```python
from build123d import *

# Parameters (mm, degrees)
F0_W     = 100
F0_H     = 100
F1_DEPTH = 100
F2_R     = 10
F3_R     = 7.3330548606
F4_DEPTH = 5
F5_R     = 7.0099311872
F5_R_2   = 5.9405048223
F6_DEPTH = 18


# Not quite as in the source:
# - a fillet or chamfer that OpenCascade refuses, or shapes differently, is made with other operations: its cross-section is extruded or revolved along the edge and cut away or added


with BuildPart() as f1:
    # F0 (on Top) → F1 (new body)
    with BuildSketch(Plane.XY):
        Rectangle(F0_W, F0_H)
    extrude(amount=F1_DEPTH)

    # F2
    f2_edges = [f1.edges().sort_by_distance(p)[0] for p in [
        (-50, -50, 50),
        (0, -50, 0),
        (50, -50, 50),
        (-50, 0, 100),
        (0, 50, 100),
        (50, 0, 100),
        (0, -50, 100),
        (-50, 0, 0),
        (-50, 50, 50),
        (0, 50, 0),
        (50, 50, 50),
        (50, 0, 0),
    ]]
    fillet(f2_edges, radius=F2_R)

    # F3 (on face) → F4 (cut)
    with BuildSketch(Plane(origin=(-50, 0, 0), x_dir=(0, -1, 0), z_dir=(-1, 0, 0))):
        with Locations((1.8755461788, 50)):
            Circle(F3_R)
    extrude(amount=-F4_DEPTH, mode=Mode.SUBTRACT)

    # F5 (on face) → F6 (cut)
    with BuildSketch(Plane.YZ.offset(50)):
        with Locations((19.523344934, 76.1831775308)):
            Circle(F5_R)
        with Locations((-10.0353639573, 45.1647788286)):
            Circle(F5_R_2)
    extrude(amount=-F6_DEPTH, mode=Mode.SUBTRACT)

    # F7: fillet of radius 7.2426406871 on 5 edges, made by hand

    # F7_s1 → F7_t2 (revolve)
    with BuildSketch(Plane.XY.offset(50)):
        with BuildLine():
            ThreePointArc((-50, -9.2086010394), (-46.3818180141, -6.5771030138), (-45, -2.3219177396))
            Line((-45, -2.3219177396), (-45, -9.2086010394))
            Line((-45, -9.2086010394), (-50, -9.2086010394))
        make_face()
    revolve(axis=Axis((-45, -1.8755461788, 50), (-1, 0, 0)))


solid = f1.part
```
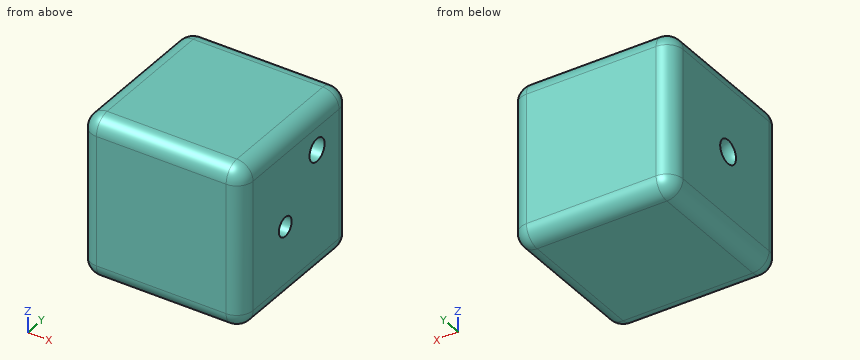
Read the model definition and answer for the solid it produces. Units are mm, in the model's axes. Give positions to 0.01 mm unless a question says otherwise; leave off trailing zeros. Order: outer loops, then holes, each group sorted by start corner. A loop starts at its lowest first (then second) coordinate and runs counter-clockwise, first axis right, second up. Notation, with made-up numbers: (49.5, 44.5) -> (53.5, 44.5) arc R30 ccw to (53.5, 71.5) -> close; hole circle Ø2 at (71.5, 69). An arc over 180 degrees is marked (long way). Write item = value, one per line.
1. A cutting plane is placed at B-B, the plane z = 73. Write down the section's boundary in (x, y).
Numbers:
outline = (-50, -40) arc R10 ccw to (-40, -50) -> (40, -50) arc R10 ccw to (50, -40) -> (50, 13.28) -> (32, 13.28) -> (32, 25.77) -> (50, 25.77) -> (50, 40) arc R10 ccw to (40, 50) -> (-40, 50) arc R10 ccw to (-50, 40) -> close
2. A cutting plane is placed at A-A, the plane y = 20. Write down the section's boundary in (x, z).
Numbers:
outline = (-50, 10) arc R10 ccw to (-40, 0) -> (40, 0) arc R10 ccw to (50, 10) -> (50, 69.19) -> (32, 69.19) -> (32, 83.18) -> (50, 83.18) -> (50, 90) arc R10 ccw to (40, 100) -> (-40, 100) arc R10 ccw to (-50, 90) -> close
3. Straight lines are drawn through the part: line 1 along Y through (x, z) = (-44.5, 79.5); line 2 along Z through (x, y) = (-15.5, -43); line 3 along X through (y, z) = (9.5, 93). For each, find the intervals that lie inside material, in ascending order.
Numbers:
line_1 = -48.93 to 48.93
line_2 = 0.46 to 99.54
line_3 = -49.54 to 49.54
